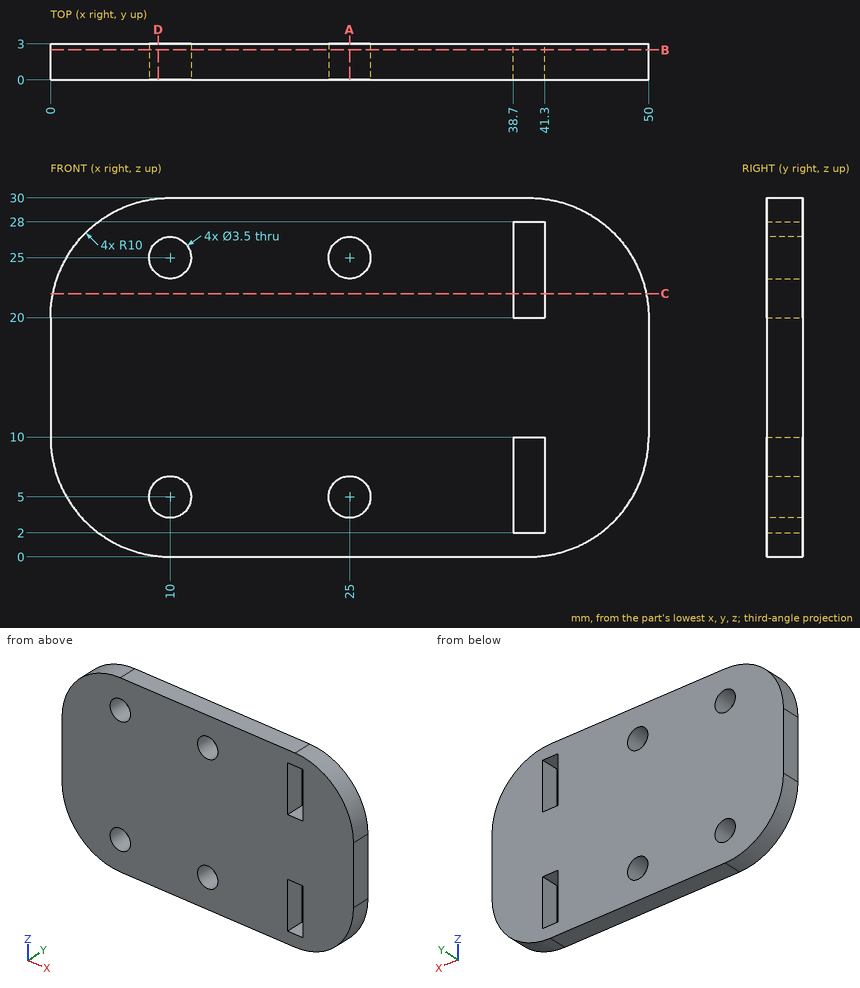
For this review, use the dimensioned drawing (mm, ordinates from the lowest corner) and the shaded views. Give positions to 0.01 mm unless a question says otherwise; leave off trailing zeros. Write each loop counter-clockwise with the first axis right and the second up, starting at its lowest first coordinate (ties: lowest second). Pieces come first, ordered by that corner, then holes. Notation, with made-up numbers: M 60.25,17 L 90.25,17 A16 ccw 90.25,26 Z; hole C 13,30.5 d6. An arc over 180 degrees is marked long. Answer as a JSON object with one key per item and string values. Group by question number.
Item 1: Consider section D-D on x = 9. Write out the cut boundary in (y, z), plus the area to 3 significant figures.
Item 2: For probe 1 along Z at (x, y) = (8.5, 0.2); probe 2 along X at (y, z) = (1.7, 5); probe 3 along Z at (x, y) = (26, 2.05), list the stretches that pass through material, from the lowest coordinate up. Write a range as [from, to].
Item 3: Consider section C-C on z = 22. Write out the cut boundary in (x, y).
Item 4: Consider section A-A on x = 25. Write out the cut boundary in (y, z), plus the area to 3 significant figures.
Item 5: For pin 1 Ø1.5 at (y, z) = (2, 24.5) entering from -X; pin 2 Ø3 at (x, z) = (25, 5) entering from -Y, all flat-tipped, find the tip position at first contact; note any pin that passes through.
Item 6: Consider section B-B on y = 2.5. Write out the cut boundary in (x, z).
Check result:
{
 "1": {"outline": "M 0,0.05 L 3,0.05 L 3,3.56 L 0,3.56 Z; M 0,6.44 L 3,6.44 L 3,23.56 L 0,23.56 Z; M 0,26.44 L 3,26.44 L 3,29.95 L 0,29.95 Z", "area": "72.5 mm^2"},
 "2": {"probe 1": "z = [0.11, 4.1], [5.9, 24.1], [25.9, 29.89]", "probe 2": "x = [1.34, 8.25], [11.75, 23.25], [26.75, 38.7], [41.3, 48.66]", "probe 3": "z = [0, 3.56], [6.44, 23.56], [26.44, 30]"},
 "3": {"outline": "M 0.2,0 L 38.7,0 L 38.7,3 L 0.2,3 Z; M 41.3,0 L 49.8,0 L 49.8,3 L 41.3,3 Z"},
 "4": {"outline": "M 0,0 L 3,0 L 3,3.25 L 0,3.25 Z; M 0,6.75 L 3,6.75 L 3,23.25 L 0,23.25 Z; M 0,26.75 L 3,26.75 L 3,30 L 0,30 Z", "area": "69.0 mm^2"},
 "5": {"pin 1": "stops at x = 0.73", "pin 2": "passes through"},
 "6": {"outline": "M 0,10 A10 ccw 10,0 L 40,0 A10 ccw 50,10 L 50,20 A10 ccw 40,30 L 10,30 A10 ccw 0,20 Z; hole C 10,5 d3.5; hole C 10,25 d3.5; hole C 25,5 d3.5; hole C 25,25 d3.5; hole M 38.7,2 L 41.3,2 L 41.3,10 L 38.7,10 Z; hole M 38.7,20 L 41.3,20 L 41.3,28 L 38.7,28 Z"}
}
